```python
from build123d import *

# Parameters (mm, degrees)
F0_R     = 101.6
F0_R_2   = 98.425
F1_DEPTH = 181.61
F0_R_3   = 95
F2_DEPTH = 177.8
F4_DEPTH = 101.601


with BuildPart() as f1:
    # F0 (on Top) → F1 (new body)
    with BuildSketch(Plane.XY):
        Circle(F0_R)
        Circle(F0_R_2, mode=Mode.SUBTRACT)
    extrude(amount=F1_DEPTH)

    # F0 (on Top) → F2 (join)
    with BuildSketch(Plane.XY):
        Circle(F0_R_2)
        Circle(F0_R_3, mode=Mode.SUBTRACT)
    extrude(amount=F2_DEPTH)

    # F3 (on Front) → F4 (cut, through all)
    with BuildSketch(Plane.XZ):
        with BuildLine():
            ThreePointArc((0, -25.4), (17.9605122421, -17.9605122421), (25.4, 0))
            ThreePointArc((25.4, 0), (-17.9605122421, 17.9605122421), (0, -25.4))
        make_face()
    extrude(amount=-F4_DEPTH, mode=Mode.SUBTRACT)


solid = f1.part
```
The listing builds one solid part. Answer for the finished solid, in the listing's coordinates (mm). A direction names the side the tool comes from. Coordinates: 2 decimals unless noted, no trailing zeros. Loops run counter-clockwise (first coordinate to the right, second up) from the corner with the lowest first, then second, coordinate; pieces in that order, holes last. Notation, with made-up numbers: M 41.5,4 L 57.5,4 A27 ccw 57.5,21 Z; hole C 51.5,69 d6. An arc over 180 degrees is marked long. Answer as CSV lines item,"result". Start each with the question number.
(1) The part is cut by section C-C (z = 143). Give the vertices of the cut face in (x, y), and give its area (3 significant figures).
(2) The part is cut by section A-A (y = 0). Give the vertices of the cut face in (x, z) (3 decimals), and give its area (3 significant figures).
(3) Find the intervals of material crossed by L1, parallel to Y at x = 0, z = 103; L2, parallel to Y at x = 0, z = 180.7 (3 decimals), in increasing order. Write a range as [from, to].
(4) The part is cut by section B-B (x = 0). Give the vertices of the cut face in (y, z) (3 decimals).
(5) The mould has two halves that part along Y. Classify faces 1 (the flat face through (-83.3, 53.2, 181.61)), 2 (the cylindrical face through (-20.59, -92.74, 87.66)), 3 (the cylindrical face through (-22.025, -99.184, 89.534)): pulls with the +Y half, pulls with the -Y half, needs draft (parallel to the pull), parting line crosses it, or undercut.
(6) For faces 4 (the flat face through (-31, -90, 0)), 5 (the cylindrical face through (0.559, 96.524, 25.394)), 6 (the flat face through (-51, 81, 177.8)), determine the directions among +Z, -Z, +X, -X, +Y, -Y from which every point of the face is accessible in a straight line to the end or side of a thin tool.
(7) Given pin 1 (1 mm diameter, centred on x = 60, z = 133.5, fed in from +Y); pin 2 (3 mm diameter, centred on x = 72, z = 161.5, fed in from +Y); pin 3 (2 mm diameter, centred on y = -35, z = 160.5, fed in from +X), each flat-ended and moving along its own axis, determine where each tip first touches the part or whether it passes through.
Determined:
1,outline,"C 0,0 d203.2; hole C 0,0 d190"
1,area,"4,080 mm2"
2,outline,"M -101.6,0 L -95,0 L -95,177.8 L -98.425,177.8 L -98.425,181.61 L -101.6,181.61 Z; M 95,0 L 101.6,0 L 101.6,181.61 L 98.425,181.61 L 98.425,177.8 L 95,177.8 Z"
2,area,"2,370 mm2"
3,L1,"[-101.6, -95], [95, 101.6]"
3,L2,"[-101.6, -98.425], [98.425, 101.6]"
4,outline,"M -101.6,0 L -95,0 L -95,177.8 L -98.425,177.8 L -98.425,181.61 L -101.6,181.61 Z; M 95,25.4 L 101.6,25.4 L 101.6,181.61 L 98.425,181.61 L 98.425,177.8 L 95,177.8 Z"
5,face 1,"needs draft"
5,face 2,"undercut"
5,face 3,"parting line crosses it"
6,face 4,"-Z, +X, -X, +Y, -Y"
6,face 5,"-Z, +Y"
6,face 6,"+Z"
7,pin 1,"y = 82.35"
7,pin 2,"y = 73.16"
7,pin 3,"x = 95.74"
